Print and shaded views of the part. All mm, measured from the part's lowest x, y and z. Give positions to 0.01 mm unless a question says otherwise; leave off trailing zeros. Write each loop counter-clockwise with the first axis right and the second up, starting at its lowest first coordinate (ties: lowest second). Pieces come first, ordered by that corner, then holes. Notation, with made-up numbers: (-13.5, 27.5) - (17.5, 27.5) arc R15 cw to (17.5, 40.5) - close; hole circle Ø9 at (55, 16.25). An arc over 180 degrees is marked (long way). Use one line per item in the form item = value. Start each with the question number.
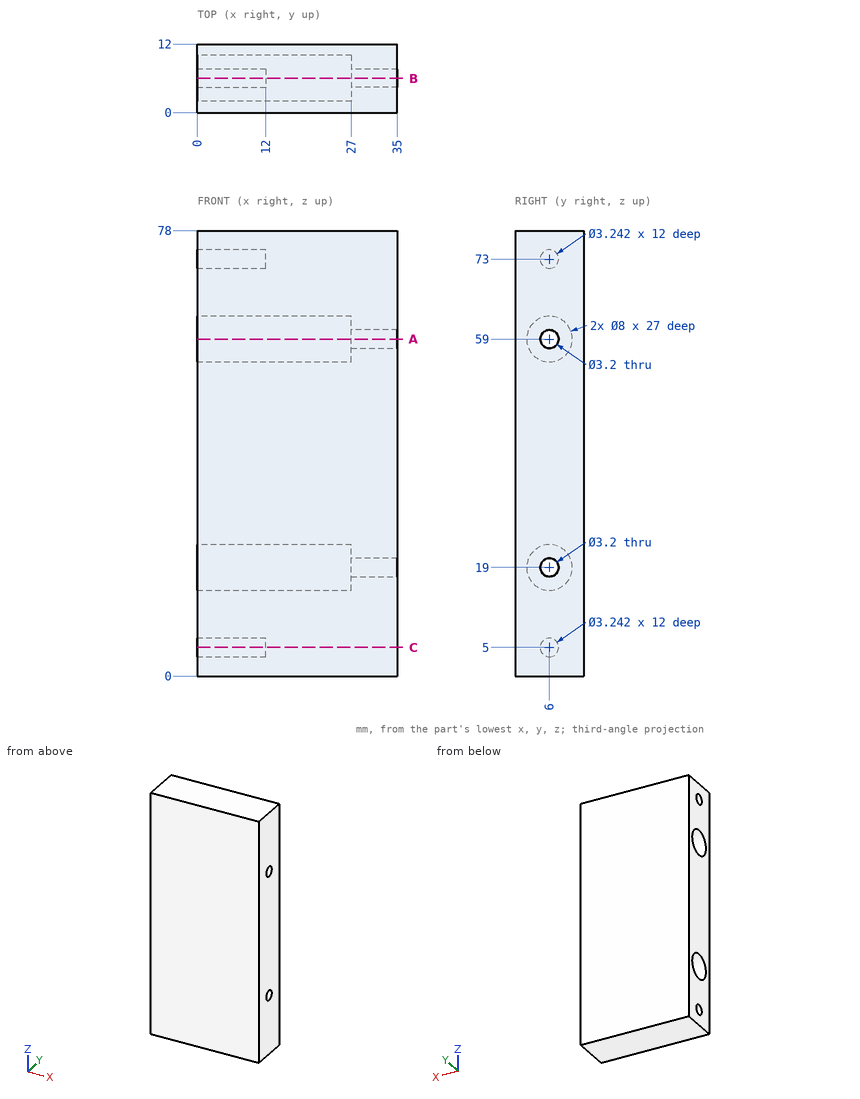
(1) Cut at B-B, the plane y = 6. Give the cut face in (x, z).
(2) Cut at C-C, the plane z = 5. Give the cut face in (x, y).
(3) Pin check, flat tips, straight feed: pin 1 Ø2.5 at (y, z) = (6, 19) entering from +X; pin 2 Ø3.5 at (y, z) = (6, 5) entering from -X; pin 3 Ø2.5 at (y, z) = (6, 60) entering from -X. Stop position of each tip, or through.
(4) Wall check: line 1 (Z direction, x = 29, y = 6); line 2 (Z direction, x = 13, y = 8.75); line 3 (Y direction, x = 32, z = 59). Give the ranges that are in metal, low to high. Write a range as from..to.
(5) Cut at A-A, the plane z = 59. Give the cut face in (x, y), then the cut area to 3 significant figures.
Solution:
q1.outline = (0, 0) - (35, 0) - (35, 17.4) - (27, 17.4) - (27, 15) - (0, 15) - (0, 6.62) - (12, 6.62) - (12, 3.38) - (0, 3.38) - close; (0, 23) - (27, 23) - (27, 20.6) - (35, 20.6) - (35, 57.4) - (27, 57.4) - (27, 55) - (0, 55) - close; (0, 63) - (27, 63) - (27, 60.6) - (35, 60.6) - (35, 78) - (0, 78) - (0, 74.62) - (12, 74.62) - (12, 71.38) - (0, 71.38) - close
q2.outline = (0, 0) - (35, 0) - (35, 12) - (0, 12) - (0, 7.62) - (12, 7.62) - (12, 4.38) - (0, 4.38) - close
q3.pin_1 = through
q3.pin_2 = 0
q3.pin_3 = 27
q4.line_1 = 0..17.4, 20.6..57.4, 60.6..78
q4.line_2 = 0..16.1, 21.9..56.1, 61.9..78
q4.line_3 = 0..4.4, 7.6..12
q5.outline = (0, 0) - (35, 0) - (35, 4.4) - (27, 4.4) - (27, 2) - (0, 2) - close; (0, 10) - (27, 10) - (27, 7.6) - (35, 7.6) - (35, 12) - (0, 12) - close
q5.area = 178 mm2
